Geometry: see drawing. Coordinates: mm, zero at the bounding-box minimum. Give positions to 0.01 mm unless a question says otherwise; leave off trailing zeros. Write each loop counter-clockwise with the first axis right and the second up, starting at its lowest first coordinate (ties: lowest second). Pieces come first, ordered by that corner, then holes. Notation, with made-up numbers: M 45,-15.75 L 70,-15.75 A29 cw 70,8.25 Z; hole C 64,33 d3. An arc over 180 degrees is marked long. Use a Markdown table: item, result. Add a question column.
1) Section C-C on z = 41. Return the cut outline in (x, y), then the cut area to 3 significant figures.
2) Section D-D on x = 23.25. Return the cut outline in (y, z).
3) Section A-A on z = 11. Return the cut outline in (x, y).
4) Pin query (flat end, axial travel): pin 1 (0.9 mm diameter, centred on y = 1.5, z = 34, fed in from +X); pin 2 (0.9 mm diameter, centred on x = 27.5, y = 1, fed in from -Z); pin 3 (1.5 mm diameter, centred on x = 17, y = 1.5, fed in from -Z). Return the tip coordinate at first contact, or that it passes through.
5) Section B-B on y = 2.25. Return the cut outline in (x, z), then the cut area to 3 significant figures.
6) Line query: line 1 (X direction, y = 0.2, z = 44); line 2 (Z direction, x = 15.25, y = 1.8); line 3 (Z direction, x = 8.5, y = 0.2). Output: solid intervals per line, ascending.
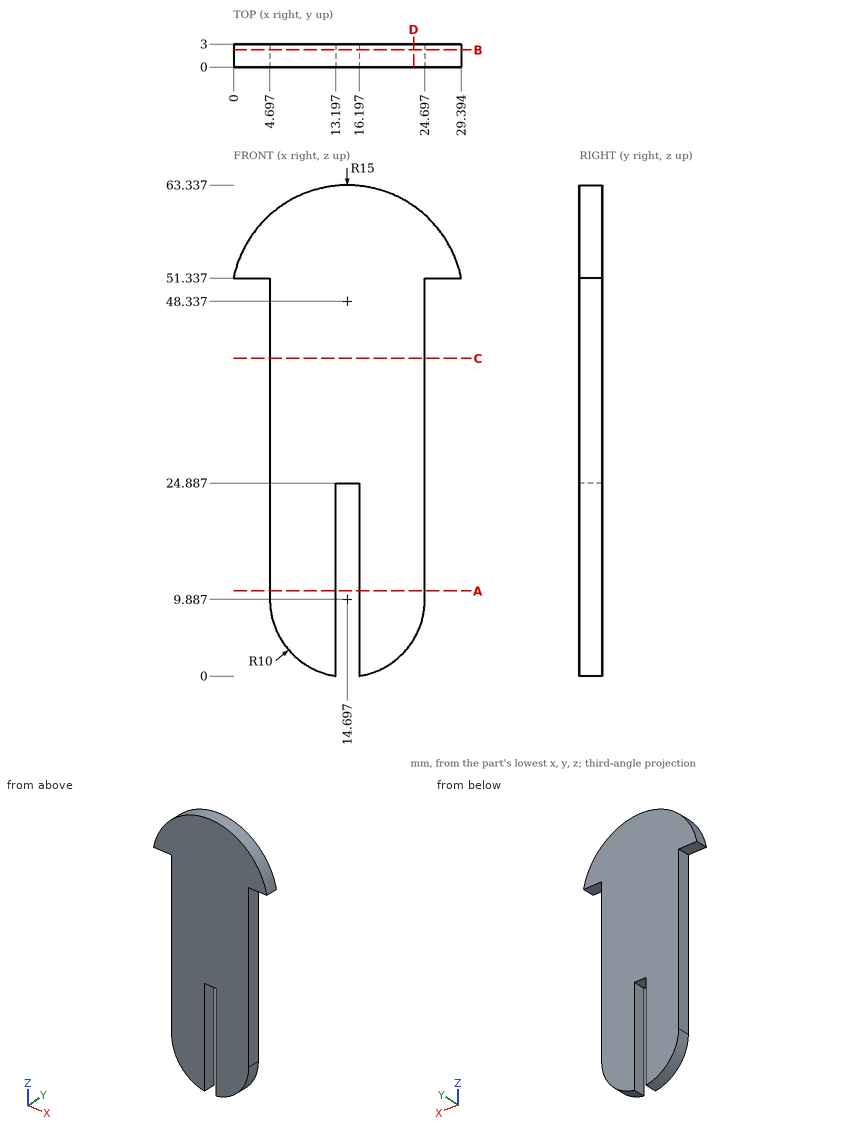
Found:
| question | item | result |
|---|---|---|
| 1 | outline | M 4.7,0 L 24.7,0 L 24.7,3 L 4.7,3 Z |
| 1 | area | 60.0 mm² |
| 2 | outline | M 0,4.71 L 3,4.71 L 3,60.66 L 0,60.66 Z |
| 3 | outline | M 4.7,0 L 13.2,0 L 13.2,3 L 4.7,3 Z; M 16.2,0 L 24.7,0 L 24.7,3 L 16.2,3 Z |
| 4 | pin 1 | x = 24.7 |
| 4 | pin 2 | z = 51.34 |
| 4 | pin 3 | z = 0.01 |
| 5 | outline | M 0,51.34 L 4.7,51.34 L 4.7,9.89 A10 ccw 13.2,0 L 13.2,24.89 L 16.2,24.89 L 16.2,0 A10 ccw 24.7,9.89 L 24.7,51.34 L 29.39,51.34 A15 ccw Z |
| 5 | area | 1,180 mm² |
| 6 | line 1 | 4.7 to 24.7 |
| 6 | line 2 | 24.89 to 63.33 |
| 6 | line 3 | 2.04 to 62 |
